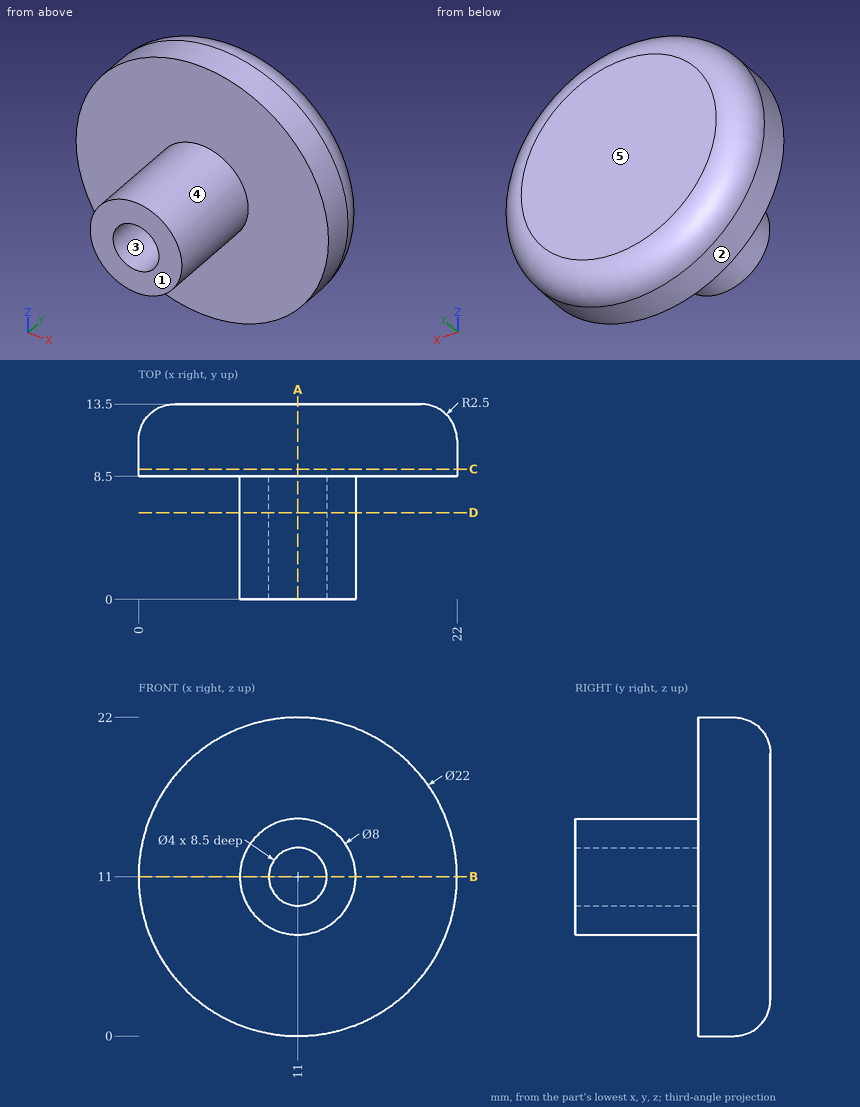
Geometry: see drawing. Coordinates: mm, zero at the bounding-box minimum. A direction names the side the tool comes from. Round coordinates to 2 decimals unless told otherwise and drop trailing zeros. Loops run counter-clockwise (first coordinate to the right, second up) from the corner with the lowest first, then second, coordinate; pieces in that order, holes last. Notation, with made-up numbers: M 49,58 L 101,58 A36 cw 101,95 Z; hole C 47,2.5 d3. An arc over 180 degrees is marked long. Use a Markdown table: item, result. Add a question column.
1. Section query A-A on x = 11. Return the cut outline in (y, z).
2. Mould query, pull axis Z, two halves, no side actions, for the marked faces 1, 2 and 3. Classes: pulls with the +Z half, pulls with the -Z half, needs draft (parallel to the pull), parting line crosses it, or undercut.
3. Section query C-C on y = 9. Return the cut outline in (x, z).
4. Reachability of the marked faces 4 and 5 from +Z, -Z, +X, -X, +Y, -Y: full face, straight path, thin tool, end or side. Return the list, or none.
5. Section query B-B on z = 11. Return the cut outline in (x, y), then the cut area to 3 significant figures.
6. Section query D-D on y = 6. Return the cut outline in (x, z), then the cut area to 3 significant figures.
7. Line query: line 1 (Z direction, x = 11, y = 1.5); line 2 (Y direction, x = 12.75, z = 4.75); line 3 (X direction, y = 7, z = 12). Output: solid intervals per line, ascending.
8. Contact query for flat-ended pins moving along their axis: P1, Ø2, axis at y = 9.5, z = 13.5, coming from the +X side; P2, Ø5, axis at y = 9.5, z = 5, coming from the -X side; P3, Ø2, axis at x = 14.5, y = 3.5, coming from the -Z side. Output: stop coordinate, or through.
Reported:
| question | item | result |
|---|---|---|
| 1 | outline | M 0,7 L 8.5,7 L 8.5,0 L 11,0 A2.5 ccw 13.5,2.5 L 13.5,19.5 A2.5 ccw 11,22 L 8.5,22 L 8.5,15 L 0,15 L 0,13 L 8.5,13 L 8.5,9 L 0,9 Z |
| 2 | face 1 | needs draft |
| 2 | face 2 | parting line crosses it |
| 2 | face 3 | undercut |
| 3 | outline | C 11,11 d22 |
| 4 | face 4 | -Y |
| 4 | face 5 | +Z, -Z, +X, -X, +Y |
| 5 | outline | M 0,8.5 L 7,8.5 L 7,0 L 9,0 L 9,8.5 L 13,8.5 L 13,0 L 15,0 L 15,8.5 L 22,8.5 L 22,11 A2.5 ccw 19.5,13.5 L 2.5,13.5 A2.5 ccw 0,11 Z |
| 5 | area | 141 mm² |
| 6 | outline | C 11,11 d8; hole C 11,11 d4 |
| 6 | area | 37.7 mm² |
| 7 | line 1 | z = 7 to 9, 13 to 15 |
| 7 | line 2 | y = 8.5 to 13.5 |
| 7 | line 3 | x = 7.13 to 9.27, 12.73 to 14.87 |
| 8 | P1 | stops at x = 21.9 |
| 8 | P2 | stops at x = 0.57 |
| 8 | P3 | stops at z = 7.88 |
